from build123d import *

# Parameters (mm, degrees)
SKETCH_3_W          = 2.5
SKETCH_3_H          = 24
EXTRUDE_1_DEPTH     = 33
FILLET_1_R          = 1
CUT_EXTRUDE_1_DEPTH = 41.880924647
SKETCH_5_W          = 2.5
SKETCH_5_H          = 3.1
CUT_EXTRUDE_2_DEPTH = 4.9
SKETCH_6_W          = 24
SKETCH_6_H          = 2.5
CUT_EXTRUDE_3_DEPTH = 1
CUT_EXTRUDE_4_DEPTH = 41.078048855
SKETCH_8_W          = 0.8
SKETCH_8_H          = 3.1
EXTRUDE_2_DEPTH     = 2.5
SKETCH_10_W         = 4.1
SKETCH_10_H         = 3.1
CUT_EXTRUDE_5_DEPTH = 41.028115119


with BuildPart() as part:
    # 草图3 → 凸台-拉伸1 (new body)
    with BuildSketch(Plane(origin=(0, 0, 0), x_dir=(0, 1, 0), z_dir=(0, 0, 1))):
        with Locations((1.25, -12)):
            Rectangle(SKETCH_3_W, SKETCH_3_H)
    extrude(amount=EXTRUDE_1_DEPTH)

    # 圆角1
    fillet_1_edges = [part.edges().sort_by_distance(p)[0] for p in [
        (24, 2.5, 16.5),
    ]]
    fillet(fillet_1_edges, radius=FILLET_1_R)

    # 草图4 → 切除-拉伸1 (cut, through all)
    with BuildSketch(Plane.XZ):
        Polygon((3, 33), (24, 31.162738066), (24, 33), align=None)
    extrude(amount=-CUT_EXTRUDE_1_DEPTH, mode=Mode.SUBTRACT)

    # 草图5 → 切除-拉伸2 (cut)
    with BuildSketch(Plane(origin=(0, 0, 0), x_dir=(0, -1, 0), z_dir=(-1, 0, 0))):
        with Locations((-1.25, 26.95)):
            Rectangle(SKETCH_5_W, SKETCH_5_H)
    extrude(amount=-CUT_EXTRUDE_2_DEPTH, mode=Mode.SUBTRACT)

    # 草图6 → 切除-拉伸3 (cut)
    with BuildSketch(Plane.XY.offset(33)):
        with Locations((12, 1.25)):
            Rectangle(SKETCH_6_W, SKETCH_6_H)
    extrude(amount=-CUT_EXTRUDE_3_DEPTH, mode=Mode.SUBTRACT)

    # 草图7 → 切除-拉伸4 (cut, through all)
    with BuildSketch(Plane.XZ):
        Polygon((24, 31.162738066), (24, 28.826114347), (6, 32), (14.430052303, 32), align=None)
    extrude(amount=-CUT_EXTRUDE_4_DEPTH, mode=Mode.SUBTRACT)

    # 草图8 → 凸台-拉伸2 (add)
    with BuildSketch(Plane(origin=(0, 2.5, 0), x_dir=(-1, 0, 0), z_dir=(0, 1, 0))):
        with Locations((-0.4, 26.95)):
            Rectangle(SKETCH_8_W, SKETCH_8_H)
    extrude(amount=-EXTRUDE_2_DEPTH)

    # 草图10 → 切除-拉伸5 (cut, through all)
    with BuildSketch(Plane(origin=(0, 1, 0), x_dir=(-1, 0, 0), z_dir=(0, -1, 0))):
        Polygon((-6, -32), (0, -32), (0, 0), (-24, 0), (-24, -28.826114347), align=None)
        with Locations((-2.85, -26.95)):
            Rectangle(SKETCH_10_W, SKETCH_10_H, mode=Mode.SUBTRACT)
    extrude(amount=-CUT_EXTRUDE_5_DEPTH, mode=Mode.SUBTRACT)


solid = part.part
The model under review builds one solid part; all positions refer to its coordinate system, in mm. A direction names the side the tool comes from. Coordinates: 2 decimals unless noted, no trailing zeros. Write each loop counter-clockwise with the first axis right and the second up, starting at its lowest first coordinate (ties: lowest second). Pieces come first, ordered by that corner, then holes. Notation, with made-up numbers: (43.25, 48) -> (50.25, 48) arc R30 ccw to (50.25, 72) -> close; hole circle Ø6 at (58.5, 14). An arc over 180 degrees is marked (long way). Answer in a Markdown table with one row per item.
1. We need section A-A, the plane x = 3.75. State the section outline as (y, z) points, and give its area (3 significant figures).
Answers below:
| item | result |
|---|---|
| outline | (0, 0) -> (1, 0) -> (1, 25.4) -> (0, 25.4) -> close; (0, 28.5) -> (1, 28.5) -> (1, 32) -> (0, 32) -> close |
| area | 28.9 mm^2 |
2. Wall thickness on probe 1 along Z at (x, y) = (3, 0.4); probe 2 along Z at (x, y) = (17.5, 0.8); probe 3 along Z at (x, y) = (10, 0.3): over which ranges is each line inside the solid? List them lowest first. Write a range as [from, to].
Answers below:
| item | result |
|---|---|
| probe 1 | z = [0, 25.4], [28.5, 32] |
| probe 2 | z = [0, 29.97] |
| probe 3 | z = [0, 31.29] |
3. We need section C-C, the plane x = 20.75. State the section outline as (y, z) points, and give its area (3 significant figures).
Answers below:
| item | result |
|---|---|
| outline | (0, 0) -> (1, 0) -> (1, 29.4) -> (0, 29.4) -> close |
| area | 29.4 mm^2 |
4. Clearance check with a flat-ended pin moving along its axis: pin 1 Ø5 at (x, z) = (8, 16) entering from -Y. State where the tip first meets the part, or that it passes through.
Answers below:
| item | result |
|---|---|
| pin 1 | stops at y = 0 |
5. For faces 4 (the flat face through (24, 0.5, 14.2)), 5 (the flat face through (4.9, 0.5, 27)), list the 3-axis set-ups (+Z, -Z, +X, -X, +Y, -Y) from which the entire face can be reached by the end or side of a thin tool; tool diameter is ignored.
Answers below:
| item | result |
|---|---|
| face 4 | +Z, -Z, +X, +Y, -Y |
| face 5 | +Y, -Y |
6. Draft analysis for pull direction Z (two halves, no side actions). For faces 1 (the flat face through (11.8, 0.5, 0)), 2 (the flat face through (2.8, 0.5, 28.5)), 3 (the flat face through (12, 1, 16)), state which applies: +Z half, -Z half, draft (parallel to the pull), parting line (faces both ways), or undercut.
Answers below:
| item | result |
|---|---|
| face 1 | -Z half |
| face 2 | undercut |
| face 3 | draft |
7. We need section B-B, the plane y = 0.6. State the section outline as (x, z) points, and give its area (3 significant figures).
Answers below:
| item | result |
|---|---|
| outline | (0, 0) -> (24, 0) -> (24, 28.83) -> (6, 32) -> (0, 32) -> close; hole (0.8, 25.4) -> (4.9, 25.4) -> (4.9, 28.5) -> (0.8, 28.5) -> close |
| area | 727 mm^2 |
8. We need section D-D, the plane x = 16.5. State the section outline as (y, z) points.
Answers below:
| item | result |
|---|---|
| outline | (0, 0) -> (1, 0) -> (1, 30.15) -> (0, 30.15) -> close |
